```python
from build123d import *

# Parameters (mm, degrees)
SKETCH1_W             = 220
SKETCH1_H             = 60
BOSS_EXTRUDE1_DEPTH   = 6.35
FILLET1_R             = 10
F_6_0MM_DOWEL_HOLE1_D = 6
F_3_0MM_DOWEL_HOLE1_D = 3
F_5_0MM_DOWEL_HOLE1_D = 5


with BuildPart() as part:
    # Sketch1 → Boss-Extrude1 (new body)
    with BuildSketch(Plane(origin=(0, 0, 0), x_dir=(1, 0, 0), z_dir=(0, 1, 0))):
        with Locations((55, 0)):
            Rectangle(SKETCH1_W, SKETCH1_H)
    extrude(amount=BOSS_EXTRUDE1_DEPTH)

    # Fillet1
    fillet1_edges = [part.edges().sort_by_distance(p)[0] for p in [
        (-55, 3.175, -30),
        (165, 3.175, -30),
        (165, 3.175, 30),
        (-55, 3.175, 30),
    ]]
    fillet(fillet1_edges, radius=FILLET1_R)

    # Ø6.0mm Dowel Hole1 (through all)
    with Locations(Plane(origin=(0, 6.35, 0), x_dir=(1, 0, 0), z_dir=(0, 1, 0))):
        with Locations((125, 0)):
            Hole(F_6_0MM_DOWEL_HOLE1_D / 2)

    # Ø3.0mm Dowel Hole1 (through all)
    with Locations(Plane(origin=(0, 6.35, 0), x_dir=(1, 0, 0), z_dir=(0, 1, 0))):
        with Locations((139, -9), (111, -9), (111, 9), (139, 9)):
            Hole(F_3_0MM_DOWEL_HOLE1_D / 2)

    # Ø5.0mm Dowel Hole1 (through all)
    with Locations(Plane(origin=(0, 6.35, 0), x_dir=(1, 0, 0), z_dir=(0, 1, 0))):
        with Locations((20, -25), (90, -25), (90, 25), (20, 25), (-40, -25), (-40, 25)):
            Hole(F_5_0MM_DOWEL_HOLE1_D / 2)


solid = part.part
```
For this review, take the finished solid that the model builds, in its own axes (mm). Coordinates: 2 decimals unless noted, no trailing zeros. Loops run counter-clockwise (first coordinate to the right, second up) from the corner with the lowest first, then second, coordinate; pieces in that order, holes last.
1. Add section C-C, the plane x = 20. Give the boundary of the cut face in (y, z), then the cut area to 4 significant figures.
2. Add section B-B, the plane y = 4. Count the separate pieces of the cut face and the enclosed holes in it, then the cut area to 3 significant figures.
3. Add section A-A, the plane x = 125. Give the boundary of the cut face in (y, z), then the cut area to 3 significant figures.
4. For line 1 (Z direction, x = 20, y = 3.25); line 2 (Z direction, x = 111, y = 2.75); line 3 (X direction, y = 4, z = 9), list the stretches that pass through material, from the lowest coordinate up.
5. Insertion check: P1, Ø1, axis at x = 142, z = 16.5, coming from the -Y side. The pin has a flat end and moves straight along its axis. Give the tip position at first contact, or say it passes through.
6. Mouldability with a two-part tool opening along X and no side actions: class faces 1 (the cylindrical face through (21.84, 3.13, -26.69)), 2 (the flat face through (-55, 3, 0)), 3 (the flat face through (54, 3, -30)) as +X half, -X half, draft (parallel to the pull), parting line (faces both ways), or undercut.
Result:
1. outline: (0, -30) - (6.35, -30) - (6.35, -27.5) - (0, -27.5) - close; (0, -22.5) - (6.35, -22.5) - (6.35, 22.5) - (0, 22.5) - close; (0, 27.5) - (6.35, 27.5) - (6.35, 30) - (0, 30) - close
1. area: 317.5 mm2
2. separate pieces: 1
2. enclosed holes: 11
2. area: 12,900 mm2
3. outline: (0, -30) - (6.35, -30) - (6.35, -3) - (0, -3) - close; (0, 3) - (6.35, 3) - (6.35, 30) - (0, 30) - close
3. area: 343 mm2
4. line 1: z = -30 to -27.5, -22.5 to 22.5, 27.5 to 30
4. line 2: z = -30 to -10.5, -7.5 to 7.5, 10.5 to 30
4. line 3: x = -55 to 109.5, 112.5 to 137.5, 140.5 to 165
5. P1: stops at y = 0
6. face 1: undercut
6. face 2: -X half
6. face 3: draft
